Could you check a few things on this model? Use its own coordinates, in mm. Round coordinates to 2 decimals unless told otherwise and drop trailing zeros. Loops run counter-clockwise (first coordinate to the right, second up) from the corner with the lowest first, then second, coordinate; pieces in that order, holes last. Notation, with made-up numbers: M 76.5,11.5 L 122.5,11.5 A15 ccw 122.5,20.5 Z; hole C 61.25,73 d8. An arc over 180 degrees is marked long. One line per item, written item: value. Start each with the question number.
Q1. Imagine slicing it at B-B (z = 0.85). Please give me the cut outline in (x, y), then the cut area to 3 significant figures.
Q2. Imagine slicing it at C-C (x = 3.5). Please give me the cut outline in (y, z), then the cut area to 3 significant figures.
Q3. Imagine slicing it at A-A (y = 0). Please give me the cut outline in (x, z).
Q4. Please list where these lines run through material, in increasing order: line 1 along Y through (x, z) = (2.5, 0.7); line 2 along X through (y, z) = (57.5, 2.25); line 3 along Y through (x, z) = (1.25, 0.6).
Q5. I'm going to push flat-ended pins straight in: pin 1 Ø5 at (x, y) = (2, 39) entering from -Z; pin 2 Ø1.5 at (y, z) = (41, 1.5) entering from +X; pin 3 Ø1.5 at (y, z) = (58.5, 2) entering from -X. Where does each tip first touch, or does it pass through?
Q6. Imagine slicing it at D-D (y = 30.5). Please give me the cut outline in (x, z), then the cut area to 3 significant figures.
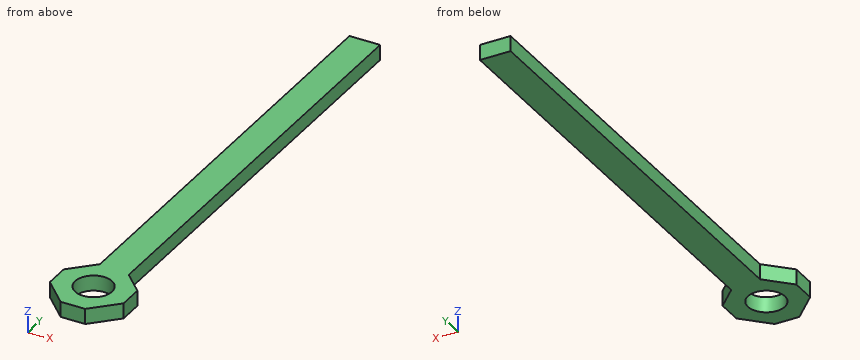
from build123d import *

# Parameters (mm, degrees)
F0_R         = 3
F0_W         = 5
F0_H         = 72
F1_DEPTH     = 2.5
F2_T1_DEPTH  = 23.0734639037
F2_T6_DEPTH  = 23.0734639037
F2_T11_DEPTH = 23.0734639037


# Not quite as in the source:
# - a fillet or chamfer that OpenCascade refuses, or shapes differently, is made with other operations: its cross-section is extruded or revolved along the edge and cut away or added


with BuildPart() as f1:
    # F0 (on Top) → F1 (new body)
    with BuildSketch(Plane.XY):
        Polygon((5, 6), (0, 6), (-3.7796038147, 6), (-3.7796038147, -6), (8.2203961853, -6), (8.2203961853, 6), align=None)
        with Locations((2.2203961853, 0)):
            Circle(F0_R, mode=Mode.SUBTRACT)
        with Locations((2.5, 42)):
            Rectangle(F0_W, F0_H)
    extrude(amount=F1_DEPTH)

    # F2: chamfer of 4 on 4 edges, made by hand

    # F2_s2 → F2_t1 (cut)
    with BuildSketch(Plane.XY.offset(-10.2867319519)):
        Polygon((4.2203961853, -6), (8.2203961853, -2), (8.2203961853, -6), align=None)
        Polygon((-3.7796038147, -2), (0.2203961853, -6), (-3.7796038147, -6), align=None)
    extrude(amount=F2_T1_DEPTH, mode=Mode.SUBTRACT)


with BuildPart() as f2_tool4:
    # F2_s5 → F2_t6 (new body)
    with BuildSketch(Plane.XY.offset(-10.2867319519)):
        Polygon((0.2203961853, 6), (-3.7796038147, 2), (-3.7796038147, 6), align=None)
    extrude(amount=F2_T6_DEPTH)

    split(bisect_by=Plane.YZ, keep=Keep.BOTTOM)


with BuildPart() as f1_1:
    add(f1.part)

    # F2_t3: cut F2_tool4
    add(f2_tool4.part, mode=Mode.SUBTRACT)


with BuildPart() as f2_tool9:
    # F2_s10 → F2_t11 (new body)
    with BuildSketch(Plane.XY.offset(-10.2867319519)):
        Polygon((4.2203961853, 6), (8.2203961853, 2), (8.2203961853, 6), align=None)
    extrude(amount=F2_T11_DEPTH)

    split(bisect_by=Plane.YZ.offset(5), keep=Keep.TOP)


with BuildPart() as f1_2:
    add(f1_1.part)

    # F2_t8: cut F2_tool9
    add(f2_tool9.part, mode=Mode.SUBTRACT)


solid = f1_2.part
Report:
1. outline: M -3.78,-2 L 0.22,-6 L 4.22,-6 L 8.22,-2 L 8.22,2 L 5,5.22 L 5,78 L 0,78 L 0,5.78 L -3.78,2 Z; hole C 2.22,0 d6
1. area: 444 mm²
2. outline: M -6,0 L -2.71,0 L -2.71,2.5 L -6,2.5 Z; M 2.71,0 L 78,0 L 78,2.5 L 2.71,2.5 Z
2. area: 196 mm²
3. outline: M -3.78,0 L -0.78,0 L -0.78,2.5 L -3.78,2.5 Z; M 5.22,0 L 8.22,0 L 8.22,2.5 L 5.22,2.5 Z
4. line 1: y = -6 to -2.99, 2.99 to 78
4. line 2: x = 0 to 5
4. line 3: y = -6 to -2.84, 2.84 to 78
5. pin 1: stops at z = 0
5. pin 2: stops at x = 5
5. pin 3: stops at x = 0
6. outline: M 0,0 L 5,0 L 5,2.5 L 0,2.5 Z
6. area: 12.5 mm²
